from build123d import *

# Parameters (mm, degrees)
F1_DEPTH = 155
F2_R     = 5.5
F3_DEPTH = 50
F4_R     = 3
F5_DEPTH = 25


with BuildPart() as f1:
    # F0 (on Front) → F1 (new body, symmetric)
    with BuildSketch(Plane.XZ):
        Polygon((35, 17.5), (35, -17.5), (-35, -17.5), (-35, 17.5), (-40, 17.5), (-40, -22.5), (40, -22.5), (40, 17.5), align=None)
    extrude(amount=F1_DEPTH, both=True)

    # F2 (on Right) → F3 (cut, symmetric)
    with BuildSketch(Plane.YZ):
        with Locations((120, -2.5)):
            Circle(F2_R)
        with Locations((-120, -2.5)):
            Circle(F2_R)
    extrude(amount=F3_DEPTH, both=True, mode=Mode.SUBTRACT)

    # F4 (on face) → F5 (cut)
    with BuildSketch(Plane.XY.offset(-17.5)):
        with Locations((-14, 145)):
            Circle(F4_R)
        with Locations((14, 145)):
            Circle(F4_R)
        with Locations((-14, 68)):
            Circle(F4_R)
        with Locations((14, 68)):
            Circle(F4_R)
        with Locations((-14, -68)):
            Circle(F4_R)
        with Locations((14, -68)):
            Circle(F4_R)
        with Locations((-14, -145)):
            Circle(F4_R)
        with Locations((14, -145)):
            Circle(F4_R)
    extrude(amount=-F5_DEPTH, mode=Mode.SUBTRACT)


solid = f1.part
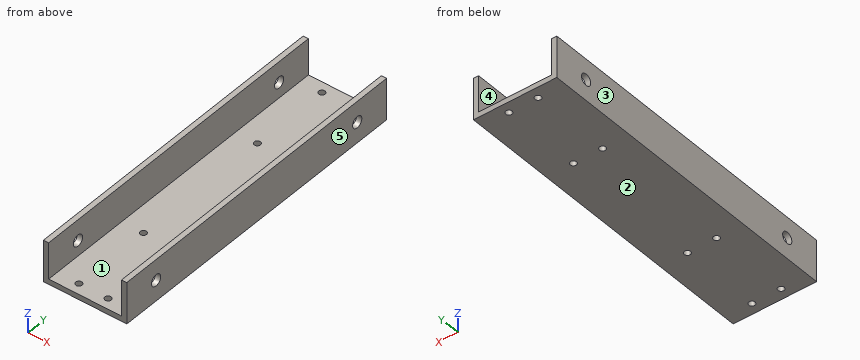
Verification items for the finished model (mm, model axes). Face numbers are marked on the shaded views. A direction names the side the tool comes from. Round coordinates to 2 decimals unless told otherwise and drop trailing zeros. Loops run counter-clockwise (first coordinate to the right, second up) from the corner with the lowest first, then second, coordinate; pieces in that order, holes last. Notation, with made-up numbers: (-11.75, 81) - (21.25, 81) arc R19 cw to (21.25, 105) - close; hole circle Ø7 at (-33.75, -36). An arc over 180 degrees is marked (long way). Use a Markdown table: item, result. Add a question column.
1. Section check A-A, the plane z = 6. Record the boundary of the cut face in (x, y), plus the area to 3 significant figures.
2. Release check for a two-part mould opening along X. For the marked faces 1, 2 and 3 record: released by +X, released by -X, zero draft, split by the parting line, or undercut.
3. Section check B-B, the plane y = 68. Record the boundary of the cut face in (x, z).
4. Thickness scan on probe 1 along X at (y, z) = (145, -18.55); probe 2 along Y at (x, z) = (14, -19); probe 3 along X at (y, z) = (-68, -10). Record the ranges inside material, lowest first. Write a range as [from, to].
5. Access from +Z, -Z, +X, -X, +Y, -Y to the whole of each face (thin tool, end or side, straight path). Record for the marked faces 4 and 5.
6. Gauge pin test, flat ends, axial feed: pin 1 (8 mm diameter, centred on x = 14, y = -68, fed in from +Z); pin 2 (9 mm diameter, centred on y = 120, z = -2.5, fed in from +X). Record the tip position at first contact, or that the pin passes through.
7. Section check D-D, the plane y = -120. Record the boundary of the cut face in (x, z), plus the area to 3 significant figures.
8. Section check C-C, the plane x = -14. Record the boundary of the cut face in (y, z), plus the area to 3 significant figures.
Checks:
| question | item | result |
|---|---|---|
| 1 | outline | (-40, -155) - (-35, -155) - (-35, 155) - (-40, 155) - close; (35, -155) - (40, -155) - (40, 155) - (35, 155) - close |
| 1 | area | 3,100 mm^2 |
| 2 | face 1 | undercut |
| 2 | face 2 | zero draft |
| 2 | face 3 | released by -X |
| 3 | outline | (-40, -22.5) - (-17, -22.5) - (-17, -17.5) - (-35, -17.5) - (-35, 17.5) - (-40, 17.5) - close; (-11, -22.5) - (11, -22.5) - (11, -17.5) - (-11, -17.5) - close; (17, -22.5) - (40, -22.5) - (40, 17.5) - (35, 17.5) - (35, -17.5) - (17, -17.5) - close |
| 4 | probe 1 | x = [-40, -17], [-11, 11], [17, 40] |
| 4 | probe 2 | y = [-155, -148], [-142, -71], [-65, 65], [71, 142], [148, 155] |
| 4 | probe 3 | x = [-40, -35], [35, 40] |
| 5 | face 4 | +Z, +Y, -Y |
| 5 | face 5 | +Z, -Z, +X, +Y, -Y |
| 6 | pin 1 | stops at z = -17.5 |
| 6 | pin 2 | passes through |
| 7 | outline | (-40, -22.5) - (40, -22.5) - (40, -8) - (35, -8) - (35, -17.5) - (-35, -17.5) - (-35, -8) - (-40, -8) - close; (-40, 3) - (-35, 3) - (-35, 17.5) - (-40, 17.5) - close; (35, 3) - (40, 3) - (40, 17.5) - (35, 17.5) - close |
| 7 | area | 640 mm^2 |
| 8 | outline | (-155, -22.5) - (-148, -22.5) - (-148, -17.5) - (-155, -17.5) - close; (-142, -22.5) - (-71, -22.5) - (-71, -17.5) - (-142, -17.5) - close; (-65, -22.5) - (65, -22.5) - (65, -17.5) - (-65, -17.5) - close; (71, -22.5) - (142, -22.5) - (142, -17.5) - (71, -17.5) - close; (148, -22.5) - (155, -22.5) - (155, -17.5) - (148, -17.5) - close |
| 8 | area | 1,430 mm^2 |
